```python
from build123d import *

# Parameters (mm, degrees)
SKETCH001_AS_DRAWN_R                 = 2.38125
EXTRUDE001_DEPTH                     = 76.2
EXTRUDE001_ONTO_SKETCH001_ROLL_ANGLE = 90
SKETCH_W                             = 88.9
SKETCH_H                             = 38.1
EXTRUDE_DEPTH                        = 438.15


with BuildPart() as extrude001:
    # Sketch001 as drawn → Extrude001 (new)
    with BuildSketch(Plane.XY):
        with Locations((44.45, 107.95)):
            Circle(SKETCH001_AS_DRAWN_R)
        with Locations((44.45, 330.2)):
            Circle(SKETCH001_AS_DRAWN_R)
    extrude(amount=-EXTRUDE001_DEPTH)


with BuildPart() as extrude001_1:
    # Extrude001 onto Sketch001 roll: moved
    add(extrude001.part.rotate(Axis((0, 0, 0), (1, 0, 0)), EXTRUDE001_ONTO_SKETCH001_ROLL_ANGLE))


with BuildPart() as extrude001_2:
    # Extrude001 onto Sketch001 placement: moved
    add(extrude001_1.part)


with BuildPart() as cut:
    # Sketch → Extrude (new body)
    with BuildSketch(Plane.XY):
        with Locations((44.45, 19.05)):
            Rectangle(SKETCH_W, SKETCH_H)
    extrude(amount=EXTRUDE_DEPTH)

    # Cut: cut Extrude001
    add(extrude001_2.part, mode=Mode.SUBTRACT)


solid = cut.part
```
Check sheet for the modelled part. Datum: model origin and axes. Units: mm. Give positions to 0.01 mm unless a question says otherwise; leave off trailing zeros. Answer in a Markdown table with one row per item.
1) Thickness scan on L1, parallel to Z at x = 44.45, y = 28.5; L2, parallel to Z at x = 44, y = 13; L3, parallel to X at y = 15, z = 330. Record the ranges inside material, lowest first. Write a range as [from, to].
Filled sheet:
| item | result |
|---|---|
| L1 | z = [0, 105.57], [110.33, 327.82], [332.58, 438.15] |
| L2 | z = [0, 105.61], [110.29, 327.86], [332.54, 438.15] |
| L3 | x = [0, 42.08], [46.82, 88.9] |
2) Gauge pin test, flat ends, axial feed: P1, Ø5.5, axis at x = 44.45, z = 330.2, coming from the -Y side; P2, Ø3, axis at x = 44.45, z = 107.95, coming from the -Y side. Record the tip position at first contact, or that the pin passes through.
Filled sheet:
| item | result |
|---|---|
| P1 | stops at y = 0 |
| P2 | passes through |
3) Release check for a two-part mould opening along X. For faces 1 (the flat face through (0, 19, 216)), 2 (the flat face through (44, 38.1, 216)), 3 (the flat face through (88.9, 19, 216)) record: +X half, -X half, draft (parallel to the pull), parting line (faces both ways), or undercut.
Filled sheet:
| item | result |
|---|---|
| face 1 | -X half |
| face 2 | draft |
| face 3 | +X half |
